Geometry check sheet. Reference: the model listing, model coordinates, mm. A direction names the side the tool comes from. Round coordinates to 2 decimals unless told otherwise and drop trailing zeros. Order: outer loops, then holes, each group sorted by start corner. A loop starts at its lowest first (then second) coordinate and runs counter-clockwise, first axis right, second up. Notation, with made-up numbers: (54, -8) -> (65, -8) arc R15 ccw to (65, 16) -> close; hole circle Ø6 at (3.25, 86). An arc over 180 degrees is marked (long way). Answer as a JSON object with one key per item and string values. Group by question number.
from build123d import *

# Parameters (mm, degrees)
SKETCH1_R             = 2.5
BOSS_EXTRUDE1_DEPTH   = 10
BOSS_EXTRUDE1_2_DEPTH = 10
BOSS_EXTRUDE2_DEPTH   = 20
FILLET1_R             = 5
SKETCH4_R             = 7.5
BOSS_EXTRUDE3_DEPTH   = 15
BOSS_EXTRUDE4_START   = 10
SKETCH5_R             = 2.5
BOSS_EXTRUDE4_DEPTH   = 10


with BuildPart() as part:
    # Sketch1 → Boss-Extrude1 (new body)
    with BuildSketch(Plane.XY):
        with Locations((90.07, -85.065581077)):
            Circle(SKETCH1_R)
    extrude(amount=-BOSS_EXTRUDE1_DEPTH)



with BuildPart() as body_2:
    # Sketch1 → Boss-Extrude1 2 (new body)
    with BuildSketch(Plane.XY):
        with Locations((40.07, -85.065581077)):
            Circle(SKETCH1_R)
    extrude(amount=-BOSS_EXTRUDE1_2_DEPTH)


with BuildPart() as part_1:
    add(part.part)

    add(body_2.part)  # Boss-Extrude2 merges body 2
    # Sketch2 → Boss-Extrude2 (add)
    with BuildSketch(Plane.XY):
        Polygon((30.07, -73.682440954), (100.07, -73.682440954), (100.07, -102.755947539), (95.194338838, -102.755947539), (95.194338838, -111.806017714), (34.945661162, -111.806017714), (34.945661162, -102.755947539), (30.07, -102.755947539), align=None)
    extrude(amount=BOSS_EXTRUDE2_DEPTH)

    # Fillet1
    # the kernel refuses this fillet: 5 mm, written as the material it takes off along each edge
    with BuildSketch(Plane(origin=(100.07, -73.682440954, -12.5), x_dir=(-1, 0, 0), z_dir=(0, 0, 1)), Plane(origin=(95.194338838, -111.806017714, -12.5), x_dir=(0, 1, 0), z_dir=(0, 0, 1))) as fillet1_piece_1:
        with BuildLine():
            CenterArc((FILLET1_R, FILLET1_R), FILLET1_R, 180, 90)
            Line((0, FILLET1_R), (-FILLET1_R * 0.02, FILLET1_R))
            Line((-FILLET1_R * 0.02, FILLET1_R), (-FILLET1_R * 0.02, -FILLET1_R * 0.02))
            Line((-FILLET1_R * 0.02, -FILLET1_R * 0.02), (FILLET1_R, -FILLET1_R * 0.02))
            Line((FILLET1_R, -FILLET1_R * 0.02), (FILLET1_R, 0))
        make_face()
    extrude(amount=45, mode=Mode.SUBTRACT)
    with BuildSketch(Plane(origin=(100.07, -102.755947539, -12.496134366), x_dir=(0, 1, 0), z_dir=(0, 0, 1))) as fillet1_piece_2:
        with BuildLine():
            CenterArc((4.998453746, 5), FILLET1_R, 181.424965019, 88.575034981)
            Line((0, 4.875661162), (-0.099969075, 4.873174386))
            ThreePointArc((-0.099969075, 4.873174386), (-0.1, 2.437830581), (-0.1, 0))
            Line((-0.1, 0), (0, -0.1))
            Line((0, -0.1), (4.998453746, -0.1))
            Line((4.998453746, -0.1), (4.998453746, 0))
        make_face()
    extrude(amount=44.992268731, mode=Mode.SUBTRACT)
    with BuildSketch(Plane(origin=(34.945661162, -111.806017714, -12.5), x_dir=(0, 1, 0), z_dir=(0, 0, 1)), Plane(origin=(30.07, -73.682440954, -12.5), x_dir=(1, 0, 0), z_dir=(0, 0, 1))) as fillet1_piece_3:
        with BuildLine():
            CenterArc((FILLET1_R, -FILLET1_R), FILLET1_R, 90, 90)
            Line((0, -FILLET1_R), (-FILLET1_R * 0.02, -FILLET1_R))
            Line((-FILLET1_R * 0.02, -FILLET1_R), (-FILLET1_R * 0.02, FILLET1_R * 0.02))
            Line((-FILLET1_R * 0.02, FILLET1_R * 0.02), (FILLET1_R, FILLET1_R * 0.02))
            Line((FILLET1_R, FILLET1_R * 0.02), (FILLET1_R, 0))
        make_face()
    extrude(amount=45, mode=Mode.SUBTRACT)
    with BuildSketch(Plane(origin=(30.07, -102.755947539, -12.496134366), x_dir=(0, 1, 0), z_dir=(0, 0, 1))) as fillet1_piece_4:
        with BuildLine():
            CenterArc((4.998453746, -5), FILLET1_R, 90, 88.575034981)
            Line((0, -4.875661162), (-0.099969075, -4.873174386))
            ThreePointArc((-0.099969075, -4.873174386), (-0.1, -2.437830581), (-0.1, 0))
            Line((-0.1, 0), (0, 0.1))
            Line((0, 0.1), (4.998453746, 0.1))
            Line((4.998453746, 0.1), (4.998453746, 0))
        make_face()
    extrude(amount=44.992268731, mode=Mode.SUBTRACT)

    # Sketch4 → Boss-Extrude3 (add)
    with BuildSketch(Plane.XZ.offset(111.806017714)):
        with Locations(Location((65.07, 10, 0), (0, 0, 90))):
            Circle(SKETCH4_R)
    extrude(amount=BOSS_EXTRUDE3_DEPTH)

    # Sketch5 → Boss-Extrude4 (add)
    with BuildSketch(Plane.XY.offset(20).offset(BOSS_EXTRUDE4_START)):
        with Locations((90.07, -85.065581077)):
            Circle(SKETCH5_R)
        with Locations((40.07, -85.065581077)):
            Circle(SKETCH5_R)
    extrude(amount=-BOSS_EXTRUDE4_DEPTH)


solid = part_1.part
Item 1: Sectioned sample at D-D, the plane z = -6. Enter the section's corners in (x, y).
Item 2: Set-up check for faces 1 (the flat face through (34.946, -105, 10)), 2 (the flat face through (95.194, -105, 10)), 3 (the flat face through (30.07, -88, 10)): record each of +Z, -Z, +X, -X, +Y, -Y from which the full face is reachable in a straight line by a thin tool's end or side.
Item 3: Sectioned sample at A-A, the plane z = 10. Enter the section's corners in (x, y).
Item 4: Sectioned sample at C-C, the plane y = -91.5. Enter the section's corners in (x, z), then the cut area to 3 significant figures.
Item 5: Sectioned sample at B-B, the plane x = 65.07. Enter the section's corners in (y, z).
Item 6: Depth check by flat-ended pin: pin 1 Ø19 at (x, y) = (62, -89.5) entering from -Z; pin 2 Ø3 at (y, z) = (-105, 5.5) entering from -X; pin 3 Ø5 at (x, z) = (49, 8.5) entering from -Y; pin 4 Ø16 at (x, z) = (77.5, 10) entering from -Y. Enter the tip coordinate at first touch or a pass-through.
Item 7: Thickness scan on L1, parallel to Z at x = 89, y = -111.5; L2, parallel to Y at x = 57, z = 7.5; L3, parallel to X at y = -103.5, z = 17. Record the ranges inside material, lowest first.
Item 8: Mould release check, pull along X, two halves, no side actions. Record for faces 4 (the cylindrical face through (72.39, -119.2, 8.37)), 5 (the flat face through (65, -126.806, 10)), 6 (the cylindrical face through (41.224, -87.284, 25.07)), 7 (the cylindrical face through (88.09, -86.59, -4.93)): pulls with the +X half, pulls with the -X half, needs draft (parallel to the pull), parting line crosses it, or undercut.
Result:
{
 "1": {"outline": "circle Ø5 at (40.07, -85.07); circle Ø5 at (90.07, -85.07)"},
 "2": {"face 1": "+Z, -Z, -X, -Y", "face 2": "+Z, -Z, +X, -Y", "face 3": "+Z, -Z, -X, +Y, -Y"},
 "3": {"outline": "(30.07, -97.76) arc R5 ccw to (34.95, -102.76) -> (34.95, -106.81) arc R5 ccw to (39.95, -111.81) -> (57.57, -111.81) -> (57.57, -126.81) -> (72.57, -126.81) -> (72.57, -111.81) -> (90.19, -111.81) arc R5 ccw to (95.19, -106.81) -> (95.19, -102.76) arc R5 ccw to (100.07, -97.76) -> (100.07, -78.68) arc R5 ccw to (95.07, -73.68) -> (35.07, -73.68) arc R5 ccw to (30.07, -78.68) -> close"},
 "4": {"outline": "(30.07, 0) -> (100.07, 0) -> (100.07, 20) -> (30.07, 20) -> close", "area": "1,400 mm2"},
 "5": {"outline": "(-126.81, 2.5) -> (-111.81, 2.5) -> (-111.81, 0) -> (-73.68, 0) -> (-73.68, 20) -> (-111.81, 20) -> (-111.81, 17.5) -> (-126.81, 17.5) -> close"},
 "6": {"pin 1": "stops at z = 0", "pin 2": "stops at x = 34.95", "pin 3": "stops at y = -111.81", "pin 4": "stops at y = -126.81"},
 "7": {"L1": "z = 0 to 20", "L2": "y = -111.81 to -73.68", "L3": "x = 34.95 to 95.19"},
 "8": {"face 4": "parting line crosses it", "face 5": "needs draft", "face 6": "undercut", "face 7": "undercut"}
}
